```python
from build123d import *

# Parameters (mm, degrees)
SKETCH1_W           = 7.25
SKETCH1_H           = 12.5
BOSS_EXTRUDE1_DEPTH = 7.4
SKETCH2_W           = 2
SKETCH2_H           = 2.700167795
SKETCH2_H_2         = 5.59966441
CUT_EXTRUDE1_DEPTH  = 8.25
SKETCH3_W           = 2.5
SKETCH3_H           = 3.5
SKETCH3_W_2         = 1
SKETCH3_H_2         = 0.331350256
BOSS_EXTRUDE2_DEPTH = 3


with BuildPart() as part:
    # Sketch1 → Boss-Extrude1 (new body)
    with BuildSketch(Plane.XY):
        with Locations((3.625, 6.25)):
            Rectangle(SKETCH1_W, SKETCH1_H)
    extrude(amount=BOSS_EXTRUDE1_DEPTH)

    # Sketch2 → Cut-Extrude1 (cut, through all)
    with BuildSketch(Plane(origin=(7.25, 0, 0), x_dir=(0, 0, -1), z_dir=(1, 0, 0))):
        with Locations((-6.4, 11.149916103)):
            Rectangle(SKETCH2_W, SKETCH2_H)
        with Locations((-6.4, 1.350083898)):
            Rectangle(SKETCH2_W, SKETCH2_H)
        with Locations((-6.4, 6.25)):
            Rectangle(SKETCH2_W, SKETCH2_H_2)
    extrude(amount=-CUT_EXTRUDE1_DEPTH, mode=Mode.SUBTRACT)

    # Sketch3 → Boss-Extrude2 (add)
    with BuildSketch(Plane(origin=(7.25, 0, 0), x_dir=(0, 0, -1), z_dir=(1, 0, 0))):
        with Locations((-2.7, 6.25)):
            Rectangle(SKETCH3_W, SKETCH3_H)
        with Locations((-2.303664878, 5.686580017)):
            Rectangle(SKETCH3_W_2, SKETCH3_H_2, mode=Mode.SUBTRACT)
        with Locations((-2.303664878, 6.813419983)):
            Rectangle(SKETCH3_W_2, SKETCH3_H_2, mode=Mode.SUBTRACT)
    extrude(amount=BOSS_EXTRUDE2_DEPTH)


solid = part.part
```
Geometry check sheet. Reference: the model listing, model coordinates, mm. A direction names the side the tool comes from. Coordinates: 2 decimals unless noted, no trailing zeros. Order: outer loops, then holes, each group sorted by start corner. A loop starts at its lowest first (then second) coordinate and runs counter-clockwise, first axis right, second up. Notation, with made-up numbers: M 38,70.25 L 68,70.25 A29 ccw 68,107.25 Z; hole C 8.25,4 d8. An arc over 180 degrees is marked long. Answer as a JSON object with one key per item and string values.
Q1. Cross-section at C-C on z = 6. Record the cut outline in (x, y), and give its area (3 significant figures).
Results are:
{"outline": "M 0,2.7 L 7.25,2.7 L 7.25,3.45 L 0,3.45 Z; M 0,9.05 L 7.25,9.05 L 7.25,9.8 L 0,9.8 Z", "area": "10.9 mm²"}
Q2. Scan lines: line 1 (Y direction, x = 6, z = 6); line 2 (Z direction, x = 1, y = 2.25); line 3 (X direction, y = 6.25, z = 4.5). Record each from-to range of solid material in increasing order.
Results are:
{"line 1": "y = 2.7 to 3.45, 9.05 to 9.8", "line 2": "z = 0 to 5.4", "line 3": "x = 0 to 7.25"}
Q3. Cross-section at A-A on x = 8.5. Record the cut outline in (y, z).
Results are:
{"outline": "M 4.5,1.45 L 8,1.45 L 8,3.95 L 4.5,3.95 Z; hole M 5.52,1.8 L 5.85,1.8 L 5.85,2.8 L 5.52,2.8 Z; hole M 6.65,1.8 L 6.98,1.8 L 6.98,2.8 L 6.65,2.8 Z"}
Q4. Cross-section at B-B on z = 3.5. Record the cut outline in (x, y), and give its area (3 significant figures).
Results are:
{"outline": "M 0,0 L 7.25,0 L 7.25,4.5 L 10.25,4.5 L 10.25,8 L 7.25,8 L 7.25,12.5 L 0,12.5 Z", "area": "101 mm²"}
Q5. Depth check by flat-ended pin: pin 1 Ø1.5 at (y, z) = (11, 2.5) entering from +X; pin 2 Ø1 at (x, z) = (3.5, 6.5) entering from +Y; pin 3 Ø1.1 at (x, z) = (8.5, 2.5) entering from +Y. Enter the tip coordinate at first touch or a pass-through.
Results are:
{"pin 1": "stops at x = 7.25", "pin 2": "stops at y = 9.8", "pin 3": "stops at y = 8"}
Q6. Release check for a two-part mould opening along Y. For faces 1 (the flat face through (4, 6, 5.4)), 2 (the flat face through (9, 8, 3)), 3 (the flat face through (4, 9.05, 6)), 4 (the flat face through (4, 6, 0)) record: released by +Y, released by -Y, zero draft, split by the parting line, or undercut.
Results are:
{"face 1": "undercut", "face 2": "released by +Y", "face 3": "undercut", "face 4": "zero draft"}
Q7. Tool access check on faces 5 (the flat face through (9, 6, 3.95)), 6 (the flat face through (4, 3.45, 6)), 7 (the flat face through (4, 11, 5.4)), 8 (the flat face through (9, 4.5, 3)), 9 (the flat face through (4, 1, 5.4)). Record the directions out of +Z, -Z, +X, -X, +Y, -Y that give a thin tool (end or side, any length) a straight path to the whole face; none if there is none.
Results are:
{"face 5": "+Z, +X, +Y, -Y", "face 6": "+Z, +X, -X", "face 7": "+Z, +X, -X, +Y", "face 8": "+Z, -Z, +X, -Y", "face 9": "+Z, +X, -X, -Y"}
Q8. Cross-section at D-D on x = 7. Record the cut outline in (y, z).
Results are:
{"outline": "M 0,0 L 12.5,0 L 12.5,5.4 L 9.8,5.4 L 9.8,7.4 L 9.05,7.4 L 9.05,5.4 L 3.45,5.4 L 3.45,7.4 L 2.7,7.4 L 2.7,5.4 L 0,5.4 Z"}
